```python
from build123d import *

# Parameters (mm, degrees)
SKETCH1_W           = 76.2
SKETCH1_H           = 31.75
BOSS_EXTRUDE1_DEPTH = 6.35
SKETCH2_W           = 19.05
SKETCH2_H           = 6.35
BOSS_EXTRUDE2_DEPTH = 6.35
CUT_EXTRUDE1_DEPTH  = 6.35
CUT_EXTRUDE4_DEPTH  = 6.35
SKETCH5_W           = 76.2
SKETCH5_H           = 6.35
BOSS_EXTRUDE3_DEPTH = 6.35
CUT_EXTRUDE5_DEPTH  = 6.35


with BuildPart() as part:
    # Sketch1 → Boss-Extrude1 (new body)
    with BuildSketch(Plane.XY):
        Rectangle(SKETCH1_W, SKETCH1_H)
    extrude(amount=BOSS_EXTRUDE1_DEPTH)

    # Sketch2 → Boss-Extrude2 (add)
    with BuildSketch(Plane.XY.offset(6.35)):
        with Locations((-6.35, 19.05)):
            Rectangle(SKETCH2_W, SKETCH2_H)
    extrude(amount=-BOSS_EXTRUDE2_DEPTH)

    # Sketch3 → Cut-Extrude1 (cut)
    with BuildSketch(Plane.XY.offset(6.35)):
        Polygon((-20.955, 11.811), (-18.923, 11.811), (-18.923, 9.779), (-20.955, 9.779), (-20.955, 5.715), (-23.495, 5.715), (-23.495, 9.779), (-25.527, 9.779), (-25.527, 11.811), (-23.495, 11.811), (-23.495, 15.875), (-20.955, 15.875), align=None)
        Polygon((8.255, 9.779), (8.255, 5.715), (10.795, 5.715), (10.795, 9.779), (12.827, 9.779), (12.827, 11.811), (10.795, 11.811), (10.795, 15.875), (8.255, 15.875), (8.255, 11.811), (6.223, 11.811), (6.223, 9.779), align=None)
    extrude(amount=-CUT_EXTRUDE1_DEPTH, mode=Mode.SUBTRACT)

    # Sketch4 → Cut-Extrude4 (cut)
    with BuildSketch(Plane.XY.offset(6.35)):
        Polygon((31.75, -9.525), (38.1, -9.525), (38.1, 9.525), (31.75, 9.525), (31.75, 1.27), (27.686, 1.27), (27.686, 3.302), (25.654, 3.302), (25.654, 1.27), (21.59, 1.27), (21.59, -1.27), (25.654, -1.27), (25.654, -3.302), (27.686, -3.302), (27.686, -1.27), (31.75, -1.27), align=None)
    extrude(amount=-CUT_EXTRUDE4_DEPTH, mode=Mode.SUBTRACT)

    # Sketch5 → Boss-Extrude3 (add)
    with BuildSketch(Plane.XY.offset(6.35)):
        with Locations((0, -19.05)):
            Rectangle(SKETCH5_W, SKETCH5_H)
    extrude(amount=-BOSS_EXTRUDE3_DEPTH)

    # Sketch6 → Cut-Extrude5 (cut)
    with BuildSketch(Plane.XY.offset(6.35)):
        Polygon((-9.525, -22.225), (9.525, -22.225), (9.525, -15.875), (1.27, -15.875), (1.27, -11.811), (3.302, -11.811), (3.302, -9.779), (1.27, -9.779), (1.27, -5.715), (-1.27, -5.715), (-1.27, -9.779), (-3.302, -9.779), (-3.302, -11.811), (-1.27, -11.811), (-1.27, -15.875), (-9.525, -15.875), align=None)
    extrude(amount=-CUT_EXTRUDE5_DEPTH, mode=Mode.SUBTRACT)


solid = part.part
```
Work out the finished part from the listing and answer in its coordinate system (mm). A direction names the side the tool comes from. Coordinates: 2 decimals unless noted, no trailing zeros. Loops run counter-clockwise (first coordinate to the right, second up) from the corner with the lowest first, then second, coordinate; pieces in that order, holes last. Notation, with made-up numbers: (55.5, 25.5) -> (107.5, 25.5) arc R22 ccw to (107.5, 58.5) -> close; hole circle Ø2 at (9.25, -1.5). An arc over 180 degrees is marked (long way). Answer as CSV lines item,"result".
Q1. A tool of negligible diameter and unlimited length cuts with its end or side. For faces 1 (the face through (24, 1.27, 3)), 2 (the face through (3.302, -11, 3)), 3 (the face through (-23.495, 14, 3)), from which of +Z, -Z, +X, -X, +Y, -Y can it reach the whole face along a straight path? Write none if from no direction.
Findings:
face 1,"+Z, -Z, +X"
face 2,"+Z, -Z"
face 3,"+Z, -Z, +Y"
Q2. The part is cut by section D-D on y = 0. Write down the section's boundary in (x, z).
Findings:
outline,"(-38.1, 0) -> (21.59, 0) -> (21.59, 6.35) -> (-38.1, 6.35) -> close"
Q3. The part is cut by section C-C on x = -7. Write down the section's boundary in (y, z) (3 decimals), and give its area (3 significant figures).
Findings:
outline,"(-15.875, 0) -> (22.225, 0) -> (22.225, 6.35) -> (-15.875, 6.35) -> close"
area,"242 mm²"
Q4. Find the intervals of material crossed by probe 1 along X at (y, z) = (9, 1.75) (3 decimals); probe 2 along X at (y, z) = (13.5, 2.5) (3 decimals); probe 3 along Y at (x, z) = (-20, 4.25) (3 decimals), in increasing order.
Findings:
probe 1,"x = -38.1 to -23.495, -20.955 to 8.255, 10.795 to 31.75"
probe 2,"x = -38.1 to -23.495, -20.955 to 8.255, 10.795 to 38.1"
probe 3,"y = -22.225 to 9.779, 11.811 to 15.875"
Q5. The part is cut by section A-A on y = 10.5. Write down the section's boundary in (x, z), and give its area (3 significant figures).
Findings:
outline,"(-38.1, 0) -> (-25.53, 0) -> (-25.53, 6.35) -> (-38.1, 6.35) -> close; (-18.92, 0) -> (6.22, 0) -> (6.22, 6.35) -> (-18.92, 6.35) -> close; (12.83, 0) -> (38.1, 0) -> (38.1, 6.35) -> (12.83, 6.35) -> close"
area,"400 mm²"
Q6. Each of these flat-tipped pins is pushed along its axis until it touches: pin 1 (2 mm diameter, centred on x = -0.5, z = 2.5, fed in from -Y) (3 decimals); pin 2 (1 mm diameter, centred on x = 12.5, z = 4, fed in from +Y) (3 decimals); pin 3 (1 mm diameter, centred on y = 0.5, z = 2, fed in from +X). Where does it stop, or does it pass through?
Findings:
pin 1,"stops at y = -15.875"
pin 2,"stops at y = 15.875"
pin 3,"stops at x = 21.59"
Q7. The part is cut by section B-B on y = -7. Write down the section's boundary in (x, z).
Findings:
outline,"(-38.1, 0) -> (-1.27, 0) -> (-1.27, 6.35) -> (-38.1, 6.35) -> close; (1.27, 0) -> (31.75, 0) -> (31.75, 6.35) -> (1.27, 6.35) -> close"
Q8. For a pull along X with two mould halves and no side action, classify faces 4 (the face through (-1, 0, 6.35)), 5 (the face through (10.795, 14, 3)), 6 (the face through (31.75, -5, 3)) as +X half, -X half, draft (parallel to the pull), parting line (faces both ways), or undercut.
Findings:
face 4,"draft"
face 5,"undercut"
face 6,"+X half"
